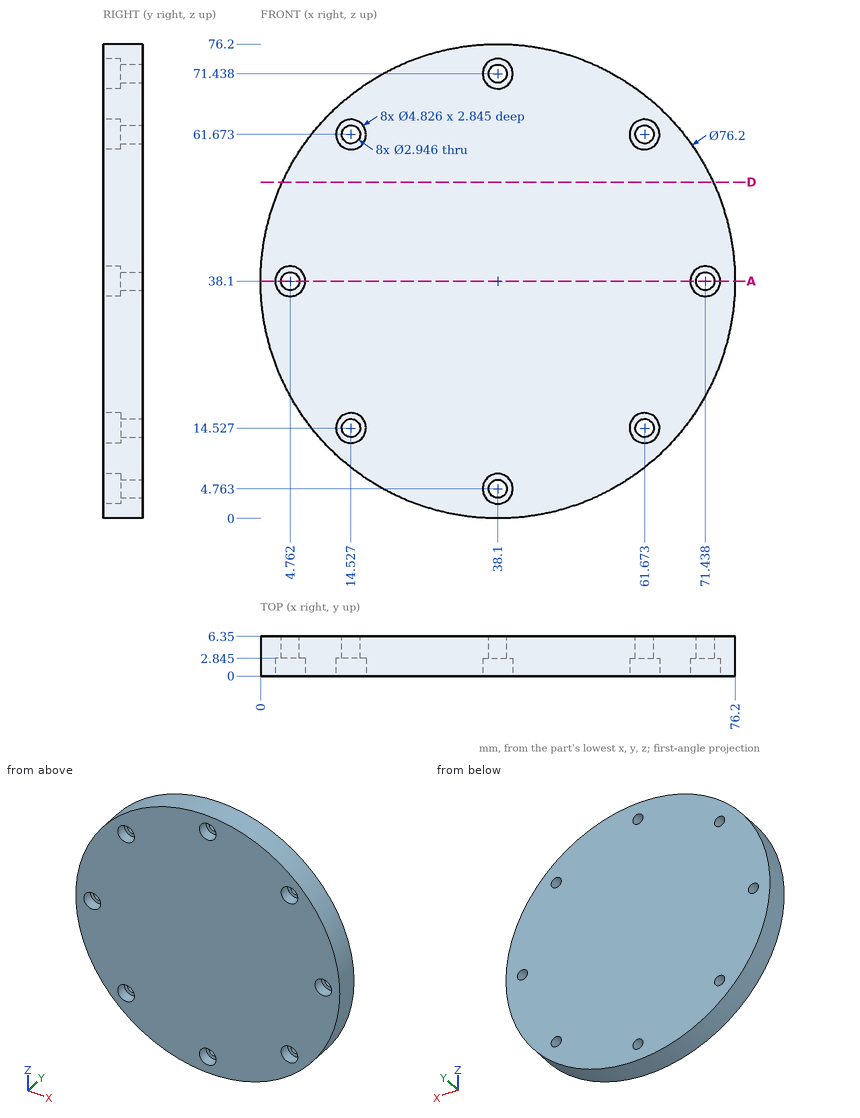
Design review of the part shown in the three views and the two pictorial views. Dimensions are in mm from the part's minimum x, y and z. Round coordinates to 2 decimals unless told otherwise and drop trailing zeros. Write each loop counter-clockwise with the first axis right and the second up, starting at its lowest first coordinate (ties: lowest second). Pieces come first, ordered by that corner, then holes.
Item 1: Clearance check with flat-ended pins moving along their axes: pin 1 Ø2 at (y, z) = (3.5, 43) entering from +X; pin 2 Ø3 at (y, z) = (4, 27.5) entering from -X; pin 3 Ø1.5 at (x, y) = (54, 3) entering from -Z. State where each tip first meets the part, or that it passes through.
Item 2: For probe 1 along X at (y, z) = (3.65, 38.1) (1 decimal); probe 2 along Z at (x, y) = (15.5, 1.75) (1 decimal); probe 3 along X at (y, z) = (2, 39) (1 decimal), list the stretches that pass through material, from the lowest coordinate up.
Item 3: We need section A-A on z = 38.1. State how many separate pieces and enclosed holes the cut face has, and give its area (3 significant figures).
Item 4: We need section D-D on z = 54. Write out the cut boundary in (x, y).
Returned:
1. pin 1: stops at x = 76
1. pin 2: stops at x = 1.1
1. pin 3: stops at z = 3.14
2. probe 1: x = 0 to 3.3, 6.2 to 70, 72.9 to 76.2
2. probe 2: z = 7.4 to 12.3, 16.7 to 59.5, 63.9 to 68.8
2. probe 3: x = 0 to 2.5, 7 to 69.2, 73.7 to 76.2
3. separate pieces: 3
3. enclosed holes: 0
3. area: 436 mm2
4. outline: (3.48, 0) - (72.72, 0) - (72.72, 6.35) - (3.48, 6.35) - close
